Can you work these out from the model? Positions are in its coordinate system, mm. Face numbers are marked on the shaded views. Give positions to 0.01 mm unless a question says otherwise; leave off trailing zeros. Write each loop counter-clockwise with the first axis right and the second up, starting at its lowest first coordinate (ties: lowest second). Pieces come first, ordered by that corner, then holes.
from build123d import *

# Parameters (mm, degrees)
F0_W     = 33
F0_H     = 33
F1_DEPTH = 166
F3_DEPTH = 100
F4_R     = 16.49999
F6_DEPTH = 50


# Not quite as in the source:
# - a fillet or chamfer is up to 0.001 mm smaller than in the source, because OpenCascade refuses the exact size


with BuildPart() as f1:
    # F0 (on Front) → F1 (new body)
    with BuildSketch(Plane.XZ):
        Rectangle(F0_W, F0_H)
    extrude(amount=F1_DEPTH)

    # F2 (on face) → F3 (cut)
    with BuildSketch(Plane.YZ.offset(16.5)):
        Polygon((-133, -16.5), (-166, 16.5), (-166, -16.5), align=None)
    extrude(amount=-F3_DEPTH, mode=Mode.SUBTRACT)

    # F4 (radius 16.5 in the source; OpenCascade refuses exactly that, so slightly less here)
    f4_edges = [f1.edges().sort_by_distance(p)[0] for p in [
        (-16.5, -83, 16.5),
        (-16.5, -66.5, -16.5),
        (16.5, -83, 16.5),
        (16.5, -66.5, -16.5),
    ]]
    fillet(f4_edges, radius=F4_R)

    # F5 (on Right) → F6 (cut, symmetric)
    with BuildSketch(Plane.YZ):
        with BuildLine():
            Line((0, -21), (0, 0))
            Line((0, 0), (0, 21))
            ThreePointArc((0, 21), (-21, 0), (0, -21))
        make_face()
    extrude(amount=F6_DEPTH, both=True, mode=Mode.SUBTRACT)


solid = f1.part
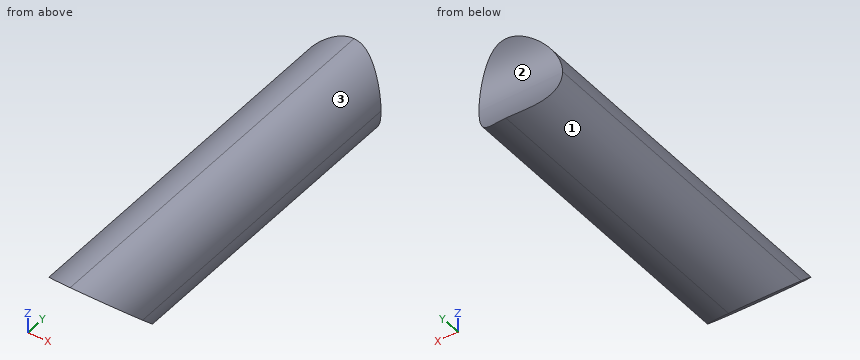
(1) Will these pins go through, and if not, where does the flat tip stop? P1, Ø10, axis at x = -1.5, z = -2, coming from the +Y side; P2, Ø3, axis at x = -9.5, z = 6, coming from the -Y side; P3, Ø5, axis at x = 10.5, y = -116, coming from the -Z side.
Returned:
P1: stops at y = -19.8
P2: stops at y = -157
P3: stops at z = -14.43
(2) Imagine slicing it at B-B, the plane x = -12. Write out the boundary of the cut face in (y, z).
Returned:
outline: (-160.82, 11.32) - (-138.18, -11.32) - (-17.68, -11.32) arc R21 cw to (-17.68, 11.32) - close
(3) Imagine slicing it at C-C, the plane z = -4. Write out the boundary of the cut face in (x, y).
Returned:
outline: (-16.01, -145.5) - (16.01, -145.5) - (16.01, -20.62) - (-16.01, -20.62) - close
(4) If I drill on L1, parallel to X at y = -76, z = -1; L2, parallel to Z at x = -13.5, y = -69.5; L3, parallel to Z at x = -13, y = -70, over which ranges is the centre line in solid material (lowest first)?
Returned:
L1: x = -16.47 to 16.47
L2: z = -9.49 to 9.49
L3: z = -10.16 to 10.16
(5) If we mould it in two halves opening along Z, with no side actions, what happens to the marked faces 1, 2 and 3? For each: +Z half, -Z half, draft (parallel to the pull), parting line (faces both ways), or undercut.
Returned:
face 1: -Z half
face 2: undercut
face 3: +Z half
